from build123d import *

# Parameters (mm, degrees)
BOSS_EXTRUDE1_DEPTH = 0.45
SKETCH3_R           = 2.2
SKETCH3_R_2         = 1.8
CUT_EXTRUDE1_DEPTH  = 0.1
SKETCH4_R           = 0.950130495
BOSS_EXTRUDE2_DEPTH = 0.05
SKETCH5_R           = 1.775413814
CUT_EXTRUDE2_DEPTH  = 0.05
SKETCH6_R           = 1.05635073
BOSS_EXTRUDE3_DEPTH = 0.08
BOSS_EXTRUDE5_DEPTH = 0.01


with BuildPart() as part:
    # Sketch1 → Boss-Extrude1 (new body)
    with BuildSketch(Plane.XY):
        with BuildLine():
            Line((-152.1, -108.5), (152.1, -108.5))
            ThreePointArc((152.1, -108.5), (155.918376618, -106.918376618), (157.5, -103.1))
            Line((157.5, -103.1), (157.5, 103.1))
            ThreePointArc((157.5, 103.1), (155.918376618, 106.918376618), (152.1, 108.5))
            Line((152.1, 108.5), (-152.1, 108.5))
            ThreePointArc((-152.1, 108.5), (-155.918376618, 106.918376618), (-157.5, 103.1))
            Line((-157.5, 103.1), (-157.5, -103.1))
            ThreePointArc((-157.5, -103.1), (-155.918376618, -106.918376618), (-152.1, -108.5))
        make_face()
    extrude(amount=BOSS_EXTRUDE1_DEPTH)

    # Sketch3 → Cut-Extrude1 (cut)
    with BuildSketch(Plane.XY.offset(0.45)):
        with Locations((0, 104.5)):
            Circle(SKETCH3_R)
        with Locations((-13.5, 104.5)):
            Circle(SKETCH3_R_2)
    extrude(amount=-CUT_EXTRUDE1_DEPTH, mode=Mode.SUBTRACT)

    # Sketch4 → Boss-Extrude2 (add)
    with BuildSketch(Plane.XY.offset(0.35)):
        with Locations((-13.5, 104.5)):
            Circle(SKETCH4_R)
    extrude(amount=BOSS_EXTRUDE2_DEPTH)

    # Sketch5 → Cut-Extrude2 (cut)
    with BuildSketch(Plane.XY.offset(0.35)):
        with Locations((0, 104.5)):
            Circle(SKETCH5_R)
    extrude(amount=-CUT_EXTRUDE2_DEPTH, mode=Mode.SUBTRACT)

    # Sketch6 → Boss-Extrude3 (add)
    with BuildSketch(Plane.XY.offset(0.3)):
        with Locations((0, 104.5)):
            Circle(SKETCH6_R)
    extrude(amount=BOSS_EXTRUDE3_DEPTH)

    # Sketch7 → Boss-Extrude5 (add)
    with BuildSketch(Plane.XY.offset(0.45)):
        with BuildLine():
            Line((157.5, 71.944818632), (156.792893219, 72.651925413))
            ThreePointArc((156.792893219, 72.651925413), (156.576120467, 72.976348762), (156.5, 73.359032194))
            Line((156.5, 73.359032194), (156.5, 97.530605069))
            ThreePointArc((156.5, 97.530605069), (156.576120467, 97.913288502), (156.792893219, 98.23771185))
            Line((156.792893219, 98.23771185), (157.5, 98.944818632))
            Line((157.5, 98.944818632), (157.5, 71.944818632))
        make_face()
        with BuildLine():
            Line((-157.5, 98.944818632), (-157.5, 71.944818632))
            Line((-157.5, 71.944818632), (-156.792893219, 72.651925413))
            ThreePointArc((-156.792893219, 72.651925413), (-156.576120467, 72.976348762), (-156.5, 73.359032194))
            Line((-156.5, 73.359032194), (-156.5, 97.530605069))
            ThreePointArc((-156.5, 97.530605069), (-156.576120467, 97.913288502), (-156.792893219, 98.23771185))
            Line((-156.792893219, 98.23771185), (-157.5, 98.944818632))
        make_face()
    extrude(amount=BOSS_EXTRUDE5_DEPTH)


solid = part.part
Verification items for the finished model (mm, model axes). Give positions to 0.01 mm unless a question says otherwise; leave off trailing zeros. Write each loop counter-clockwise with the first axis right and the second up, starting at its lowest first coordinate (ties: lowest second). Pieces come first, ordered by that corner, then holes.
(1) Gauge pin test, flat ends, axial feed: pin 1 (3.5 mm diameter, centred on x = 0, y = 104.5, fed in from +Z); pin 2 (4 mm diameter, centred on x = 68.5, y = -54, fed in from +Z); pin 3 (3 mm diameter, centred on x = -14.5, y = 21, fed in from -Z). Record the tip position at first contact, or that the pin passes through.
(2) Cross-section at B-B (x = 11.5). Enter the section's corners in (y, z).
(3) Cross-section at A-A (y = -36). Enter the section's corners in (x, z).
(4) Material ranges on line 1 (Z direction, x = 90, y = 18), recorded low to high.
Worked out:
1. pin 1: stops at z = 0.38
1. pin 2: stops at z = 0.45
1. pin 3: stops at z = 0
2. outline: (-108.5, 0) - (108.5, 0) - (108.5, 0.45) - (-108.5, 0.45) - close
3. outline: (-157.5, 0) - (157.5, 0) - (157.5, 0.45) - (-157.5, 0.45) - close
4. line 1: z = 0 to 0.45
